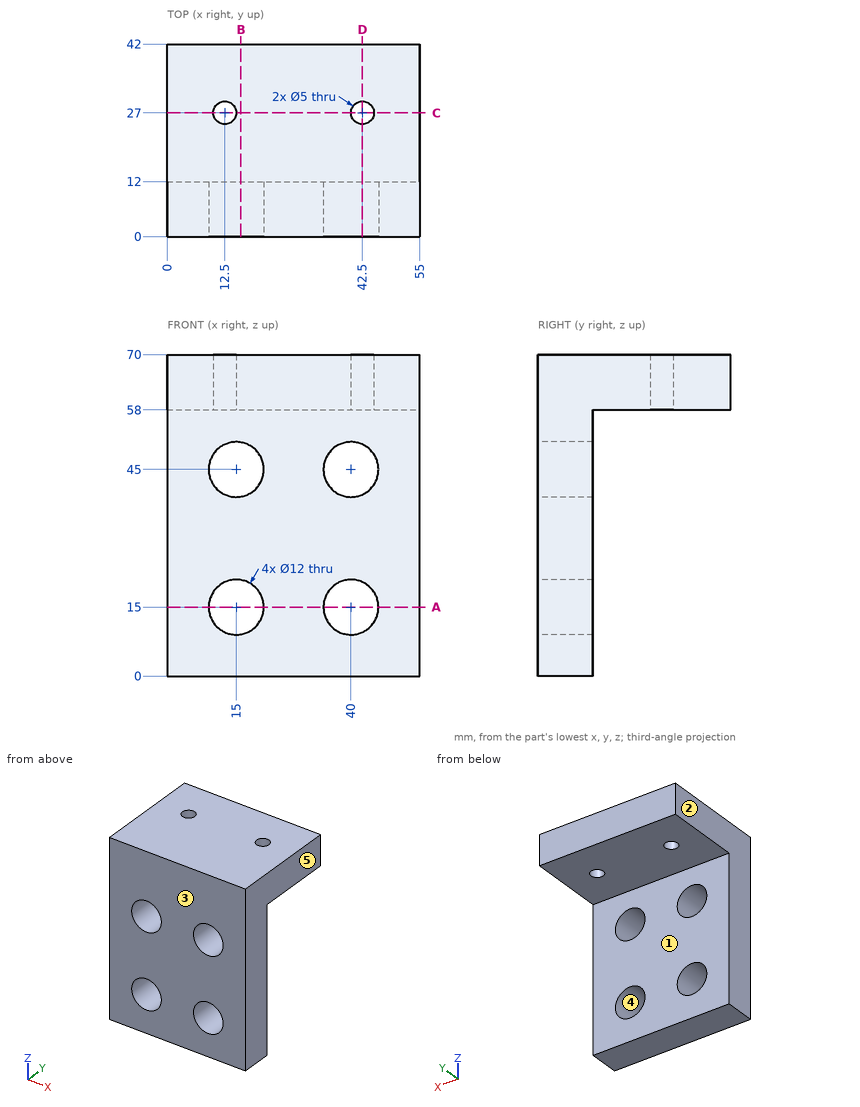
Can you work these out from the drawing? Everything is in mm from the part's minimum corner. A direction names the side the tool comes from. Give positions to 0.01 mm unless a question says otherwise; leave off trailing zeros. Order: outer loops, then holes, each group sorted by start corner. A loop starts at its lowest first (then second) coordinate and runs counter-clockwise, first axis right, second up.
1. Suppose I cut it at D-D (x = 42.5). List the corners of the cut face in (y, z) for me.
2. Suppose I cut it at C-C (y = 27). List the corners of the cut face in (x, z) for me.
3. I need wall thicknesses on L1, parallel to Z at x = 15, y = 9; L2, parallel to Z at x = 13.5, y = 6; L3, parallel to Z at x = 14.5, y = 16.5. Which ranges of each line are inside material? Lowest first, please.
4. Will these pins go through, and if not, where does the flat tip stop? P1, Ø16.5, axis at x = 21.5, z = 39, coming from the +Y side; P2, Ø8, axis at x = 42.5, y = 27, coming from the -Z side.
5. We'd pull the mould along X, two halves only. Please class the marked faces 3, 4 and 5: pulls with the +X half, pulls with the -X half, needs draft (parallel to the pull), parting line crosses it, or undercut.
6. Suppose I cut it at B-B (x = 16). List the corners of the cut face in (y, z) for me.
7. Suppose I cut it at A-A (z = 15). List the corners of the cut face in (x, y) for me, plus the area to 3 significant figures.
8. For the marked faces 1 and 2, which set-ups out of +Z, -Z, +X, -X, +Y, -Y let a thin tool reach every point of the face, with its end or its side?
Solved:
1. outline: (0, 0) - (12, 0) - (12, 9.55) - (0, 9.55) - close; (0, 20.45) - (12, 20.45) - (12, 39.55) - (0, 39.55) - close; (0, 50.45) - (12, 50.45) - (12, 58) - (24.5, 58) - (24.5, 70) - (0, 70) - close; (29.5, 58) - (42, 58) - (42, 70) - (29.5, 70) - close
2. outline: (0, 58) - (10, 58) - (10, 70) - (0, 70) - close; (15, 58) - (40, 58) - (40, 70) - (15, 70) - close; (45, 58) - (55, 58) - (55, 70) - (45, 70) - close
3. L1: z = 0 to 9, 21 to 39, 51 to 70
3. L2: z = 0 to 9.19, 20.81 to 39.19, 50.81 to 70
3. L3: z = 58 to 70
4. P1: stops at y = 12
4. P2: stops at z = 58
5. face 3: needs draft
5. face 4: undercut
5. face 5: pulls with the +X half
6. outline: (0, 0) - (12, 0) - (12, 9.08) - (0, 9.08) - close; (0, 20.92) - (12, 20.92) - (12, 39.08) - (0, 39.08) - close; (0, 50.92) - (12, 50.92) - (12, 58) - (42, 58) - (42, 70) - (0, 70) - close
7. outline: (0, 0) - (9, 0) - (9, 12) - (0, 12) - close; (21, 0) - (34, 0) - (34, 12) - (21, 12) - close; (46, 0) - (55, 0) - (55, 12) - (46, 12) - close
7. area: 372 mm2
8. face 1: -Z, +X, -X, +Y
8. face 2: +Z, -Z, -X, +Y, -Y
